Work out the finished part from the listing and answer in its coordinate system (mm). A direction names the side the tool comes from. Round coordinates to 2 decimals unless told otherwise and drop trailing zeros. Loops run counter-clockwise (first coordinate to the right, second up) from the corner with the lowest first, then second, coordinate; pieces in that order, holes last. Notation, with made-up numbers: (-25, 34.5) - (15, 34.5) arc R17 cw to (15, 61.5) - close; hole circle Ø10 at (-4.5, 47.25). An arc over 180 degrees is marked (long way). Return JSON: item names as keys, results as strings.
from build123d import *

# Parameters (mm, degrees)
F0_R     = 11
F0_R_2   = 10
F1_DEPTH = 24
F0_R_3   = 15
F2_DEPTH = 2
F3_R     = 1


with BuildPart() as f1:
    # F0 (on Top) → F1 (new body)
    with BuildSketch(Plane.XY):
        Circle(F0_R)
        Circle(F0_R_2, mode=Mode.SUBTRACT)
    extrude(amount=-F1_DEPTH)

    # F0 (on Top) → F2 (join)
    with BuildSketch(Plane.XY):
        Circle(F0_R_3)
        Circle(F0_R, mode=Mode.SUBTRACT)
        Circle(F0_R)
        Circle(F0_R_2, mode=Mode.SUBTRACT)
    extrude(amount=F2_DEPTH)

    # F3
    f3_edges = [f1.edges().sort_by_distance(p)[0] for p in [
        (-15, 0, 2),
        (-10, 0, 2),
    ]]
    fillet(f3_edges, radius=F3_R)


solid = f1.part
1) Flat-ended cylindrical pins translate along their axes: pin 1 (8 mm diameter, centred on x = -5, z = -12, fed in from -Y); pin 2 (5 mm diameter, centred on y = 0.5, z = -11, fed in from +X); pin 3 (1 mm diameter, centred on y = 9.5, z = -7.5, fed in from +X). Find the tip coordinate at first contact, or state that the pin passes through.
Verdict:
{"pin 1": "stops at y = -10.95", "pin 2": "stops at x = 11", "pin 3": "stops at x = 6.32"}
2) Determine the mould class of faces 1 (the cylindrical face through (-2.38, -10.74, -11.83)), 2 (the flat face through (6.2, -9.3, 2)), 3 (the cylindrical face through (-2.17, -9.76, -11.68)) for opening direction X: pulls with the +X half, pulls with the -X half, needs draft (parallel to the pull), parting line crosses it, or undercut.
Verdict:
{"face 1": "parting line crosses it", "face 2": "needs draft", "face 3": "undercut"}
3) A tool of negligible diameter and unlimited length cuts with its end or side. For faces 4 (the cylindrical face through (-14.985, 0.66, 0.493)), 5 (the flat face through (-5, 10, 0)), from which of +Z, -Z, +X, -X, +Y, -Y can it reach the whole face along a straight path? Write none if from no direction.
Verdict:
{"face 4": "+Z, -Z", "face 5": "-Z"}
4) Find the intervals of material crossed by L1, parallel to Y at x = 0, z = -12; L2, parallel to Z at x = 10.75, y = -1.5; L3, parallel to Y at x = -3, z = -21.5, in increasing order.
Verdict:
{"L1": "y = -11 to -10, 10 to 11", "L2": "z = -24 to 1.99", "L3": "y = -10.58 to -9.54, 9.54 to 10.58"}
5) Section A-A (y = 0) is taken. Give the vertices of the cut face in (x, z).
Verdict:
{"outline": "(-15, 0) - (-11, 0) - (-11, -24) - (-10, -24) - (-10, 1) arc R1 ccw to (-11, 2) - (-14, 2) arc R1 ccw to (-15, 1) - close; (10, -24) - (11, -24) - (11, 0) - (15, 0) - (15, 1) arc R1 ccw to (14, 2) - (11, 2) arc R1 ccw to (10, 1) - close"}
6) Section C-C (z = -16) is taken. Give the vertices of the cut face in (x, y), and give its area (3 significant figures).
Verdict:
{"outline": "circle Ø22 at (0, 0); hole circle Ø20 at (0, 0)", "area": "66.0 mm2"}
